Build history of the part. All positions in model axes, mm. Face numbers are marked on the shaded views. A direction names the side the tool comes from. Round coordinates to 2 decimals unless told otherwise and drop trailing zeros. Loops run counter-clockwise (first coordinate to the right, second up) from the corner with the lowest first, then second, coordinate; pieces in that order, holes last. Notation, with made-up numbers: M 25.25,78 L 36.25,78 A25 ccw 36.25,114 Z; hole C -21.5,43 d3. An arc over 180 degrees is marked long. One line per item, written item: value.
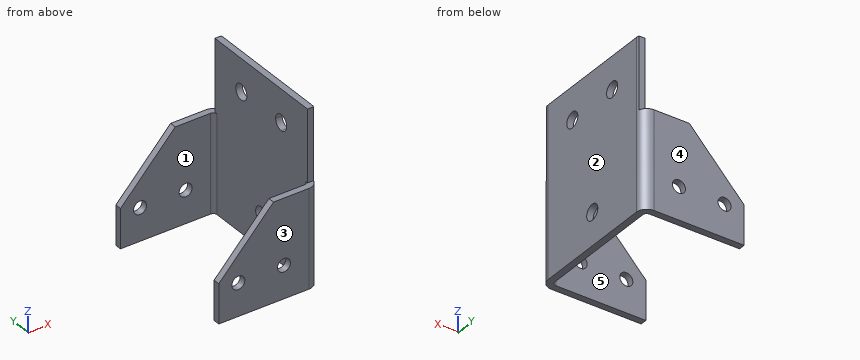
```python
from build123d import *

# Parameters (mm, degrees)
F1_DEPTH  = 130
F3_DEPTH  = 25
F5_DEPTH  = 25
F6_R      = 5
F7_DEPTH  = 200
F8_R      = 6
F9_DEPTH  = 25
F11_DEPTH = 55
F12_R     = 6
F13_DEPTH = 25


with BuildPart() as f1:
    # F0 (on Top) → F1 (new body)
    with BuildSketch(Plane.XY):
        with BuildLine():
            Line((69, 0), (0, 0))
            Line((0, 0), (0, -5))
            Line((0, -5), (69, -5))
            ThreePointArc((69, -5), (71.1213203436, -5.8786796564), (72, -8))
            Line((72, -8), (72, -32.9701863229))
            Line((72, -32.9701863229), (72, -103))
            ThreePointArc((72, -103), (71.1213203436, -105.1213203436), (69, -106))
            Line((69, -106), (0, -106))
            Line((0, -106), (0, -111))
            Line((0, -111), (69, -111))
            ThreePointArc((69, -111), (74.6568542495, -108.6568542495), (77, -103))
            Line((77, -103), (77, -8))
            ThreePointArc((77, -8), (74.6568542495, -2.3431457505), (69, 0))
        make_face()
    extrude(amount=F1_DEPTH)

    # F2 (on face) → F3 (cut)
    with BuildSketch(Plane(origin=(0, 0, 0), x_dir=(-1, 0, 0), z_dir=(0, 1, 0))):
        Polygon((0, 30), (0, 130), (-72, 130), (-72, 75), (-42, 75), align=None)
    extrude(amount=-F3_DEPTH, mode=Mode.SUBTRACT)

    # F4 (on face) → F5 (cut)
    with BuildSketch(Plane.XZ.offset(111)):
        Polygon((72, 130), (0, 130), (0, 75), (0, 30), (42, 75), (72, 75), align=None)
    extrude(amount=-F5_DEPTH, mode=Mode.SUBTRACT)

    # F6 (on face) → F7 (cut)
    with BuildSketch(Plane(origin=(0, 0, 0), x_dir=(-1, 0, 0), z_dir=(0, 1, 0))):
        with Locations((-15, 25)):
            Circle(F6_R)
        with Locations((-50, 25)):
            Circle(F6_R)
    extrude(amount=-F7_DEPTH, mode=Mode.SUBTRACT)

    # F8 (on face) → F9 (cut)
    with BuildSketch(Plane.YZ.offset(77)):
        with Locations((-55.5, 25)):
            Circle(F8_R)
    extrude(amount=-F9_DEPTH, mode=Mode.SUBTRACT)

    # F10 (on face) → F11 (cut)
    with BuildSketch(Plane.XY.offset(130)):
        with BuildLine():
            Line((72, -5.5838015129), (76.6264005187, -5.5838015129))
            ThreePointArc((76.6264005187, -5.5838015129), (74.8719755616, -2.5667778433), (72, -0.5838015129))
            Line((72, -0.5838015129), (72, -5.5838015129))
        make_face()
        with BuildLine():
            ThreePointArc((72, -110.4161984871), (74.8719755616, -108.4332221567), (76.6264005187, -105.4161984871))
            Line((76.6264005187, -105.4161984871), (72, -105.4161984871))
            Line((72, -105.4161984871), (72, -110.4161984871))
        make_face()
    extrude(amount=-F11_DEPTH, mode=Mode.SUBTRACT)

    # F12 (on face) → F13 (cut)
    with BuildSketch(Plane.YZ.offset(77)):
        with BuildLine():
            ThreePointArc((-77, 99), (-72.7573593129, 100.7573593129), (-71, 105))
            ThreePointArc((-71, 105), (-81.2426406871, 109.2426406871), (-77, 99))
        make_face()
        with Locations((-34, 105)):
            Circle(F12_R)
    extrude(amount=-F13_DEPTH, mode=Mode.SUBTRACT)


solid = f1.part
```
Item 1: Drop flat-ended pins along their axis: P1, Ø9, axis at x = 61, y = -107.5, coming from the +Z side; P2, Ø19, axis at y = -77, z = 105, coming from the -X side; P3, Ø2.5, axis at x = 74.5, z = 103.5, coming from the +Y side. Give the stop position or say it passes through.
Check values:
P1: stops at z = 75
P2: stops at x = 72
P3: stops at y = -5.58
Item 2: Slice it at A-A, the plane z = 25. Give the number of separate pieces and of enclosed holes in the cut face, and give its area (3 significant figures).
Check values:
separate pieces: 6
enclosed holes: 0
area: 991 mm2
Item 3: Slice it at C-C, the plane y = -55.5. Give the cut face in (x, z), and give its area (3 significant figures).
Check values:
outline: M 72,0 L 77,0 L 77,19 L 72,19 Z; M 72,31 L 77,31 L 77,130 L 72,130 Z
area: 590 mm2
Item 4: Wall check: line 1 along Y through (x, z) = (64, 40); line 2 along X through (y, z) = (-33.5, 36.5); line 3 along Z through (x, y) = (15, -2.3). Give the ranges that are in metal, low to high.
Check values:
line 1: y = -111 to -106, -5 to 0
line 2: x = 72 to 77
line 3: z = 0 to 20, 30 to 46.07
Item 5: Pull direction Y, two halves, no side cores. Call the marked faces 1, 2 and 3: pulls with the +Y half, pulls with the -Y half, needs draft (parallel to the pull), parting line crosses it, or undercut.
Check values:
face 1: undercut
face 2: needs draft
face 3: pulls with the -Y half
Item 6: Slice it at D-D, the plane x = 37. Give the cut face in (y, z), and give its area (3 significant figures).
Check values:
outline: M -111,0 L -106,0 L -106,69.64 L -111,69.64 Z; M -5,0 L 0,0 L 0,69.64 L -5,69.64 Z
area: 696 mm2
Item 7: Slice it at B-B, the plane x = 50. Give the cut face in (y, z).
Check values:
outline: M -111,0 L -106,0 L -106,20 L -111,20 Z; M -111,30 L -106,30 L -106,75 L -111,75 Z; M -5,0 L 0,0 L 0,20 L -5,20 Z; M -5,30 L 0,30 L 0,75 L -5,75 Z
Item 8: Which spindle directions (+Z, -Z, +X, -X, +Y, -Y) get a long thin tool onto all of the face, cutting with end or side? Do the marked faces 4 and 5. Say none if no direction does.
Check values:
face 4: +Z, -Z, +X, -X, +Y
face 5: +Z, -Z, -X
